Design review of the part built by this model. Coordinates are the model's own, in mm. A direction names the side the tool comes from. Give positions to 0.01 mm unless a question says otherwise; leave off trailing zeros. Write each loop counter-clockwise with the first axis right and the second up, starting at its lowest first coordinate (ties: lowest second). Pieces come first, ordered by that corner, then holes.
Autodesk Inventor part; units mm, degrees
ref_plane "YZ Plane" through (0, 0, 0) normal (1, 0, 0) x (0, 1, 0)
ref_plane "XZ Plane" through (0, 0, 0) normal (0, 1, 0) x (-1, 0, 0)
ref_plane "XY Plane" through (0, 0, 0) normal (0, 0, 1) x (1, 0, 0)
sketch "Sketch1" plane through (0, 0, 0) normal (0, 0, 1) x (1, 0, 0)
  line L0 (-30, -30) -> (30, -30)
  line L1 (30, -30) -> (30, 30)
  line L2 (30, 30) -> (-30, 30)
  line L3 (-30, 30) -> (-30, -30)
  line L4 (-30, -30) -> (30, 30) construction
  line L5 (30, -30) -> (-30, 30) construction
  point P0 (0, 0)
  dimension "d0" = 60
  dimension "d1" = 60
extrude "Main Block" add sketch "Sketch1" along normal blind 60
sketch "Sketch2" plane through (-30, 30, 0) normal (0, 1, 0) x (1, 0, 0)
  line L0 (0, -60) -> (60, -60) construction
  line L1 (0, 0) -> (60, 0) construction
  line L2 (60, -60) -> (0, 0) construction
  line L3 (51.25, -51.25) -> (8.75, -51.25)
  line L4 (8.75, -51.25) -> (8.75, -8.75)
  line L5 (8.75, -8.75) -> (51.25, -8.75)
  line L6 (51.25, -8.75) -> (51.25, -51.25)
  line L7 (51.25, -51.25) -> (8.75, -8.75) construction
  line L8 (8.75, -51.25) -> (51.25, -8.75) construction
  line L9 (30, -30) -> (30, -51.25) construction
  point P0 (30, 0)
  dimension "d4" = 42.5
  dimension "d5" = 42.5
extrude "Motor Void" cut sketch "Sketch2" against normal blind 58
sketch "Sketch3" plane through (-30, 30, 0) normal (0, 1, 0) x (1, 0, 0)
  line L0 (30, 0) -> (30, -8.75) construction
  line L1 (8.75, -8.75) -> (51.25, -8.75) construction
  line L2 (38.25, 0.125) -> (21.75, 0.125)
  line L3 (21.75, 0.125) -> (21.75, -8.875)
  line L4 (21.75, -8.875) -> (38.25, -8.875)
  line L5 (38.25, -8.875) -> (38.25, 0.125)
  line L6 (38.25, 0.125) -> (21.75, -8.875) construction
  line L7 (21.75, 0.125) -> (38.25, -8.875) construction
  point P0 (30, -4.375)
  dimension "d30" = 16.5
  dimension "d31" = 9
extrude "Cable Void" cut sketch "Sketch3" against normal blind 41
sketch "Sketch4" plane through (-30, -30, 0) normal (0, -1, 0) x (1, 0, 0)
  line L0 (0, 0) -> (0, 60) construction
  line L1 (60, 60) -> (0, 60) construction
  line L2 (0, 0) -> (60, 60) construction
  circle A0 centre (30, 30) radius 11
  point P0 (30, 0)
  dimension "d12" = 22
extrude "Raised Void" cut sketch "Sketch4" against normal blind 2
sketch "Sketch6" plane through (-30, -30, 0) normal (-1, 0, 0) x (0, 0, 1)
  line L0 (60, 0) -> (60, 60) construction
  line L1 (60, 60) -> (60, 55) construction
  line L2 (60, 55) -> (55, 55) construction
  line L3 (60, 0) -> (60, 5) construction
  line L4 (60, 5) -> (55, 5) construction
  line L5 (0, 0) -> (5, 0) construction
  line L6 (0, 0) -> (60, 0) construction
  line L7 (5, 0) -> (5, 5) construction
  line L8 (0, 60) -> (0, 0) construction
  line L9 (0, 60) -> (5, 60) construction
  line L10 (0, 60) -> (60, 60) construction
  line L11 (5, 60) -> (5, 55) construction
  circle A0 centre (55, 55) radius 1.5
  circle A1 centre (55, 5) radius 1.5
  circle A2 centre (5, 5) radius 1.5
  circle A3 centre (5, 55) radius 1.5
  point P0 (0, 30)
  dimension "d32" = 5
  dimension "d33" = 5
  dimension "d34" = 5
  dimension "d35" = 5
  dimension "d36" = 5
  dimension "d37" = 5
  dimension "d38" = 5
  dimension "d39" = 5
  dimension "d40" = 3
  dimension "d41" = 3
  dimension "d42" = 3
  dimension "d43" = 3
extrude "Holes" cut sketch "Sketch6" against normal blind 60
fillet "Cleaning it up" radius 5 5 edges at (0, 30, 60) (0, -30, 60) (19.125, 30, 0) (-19.125, 30, 0) (0, -30, 0)
equation "\"d4\" = d5"
properties part number "60x60Motor"
(1) Consider section D-D, the plane y = -4.5. Give the boundary of the cut face in (x, z).
Resolved:
outline: (-30, 0) - (-8.25, 0) - (-8.25, 8.75) - (-21.25, 8.75) - (-21.25, 51.25) - (21.25, 51.25) - (21.25, 8.75) - (8.25, 8.75) - (8.25, 0) - (30, 0) - (30, 60) - (-30, 60) - close
(2) Consider section A-A, the plane x = 19. Give the boundary of the cut face in (y, z).
Resolved:
outline: (-30, 5) arc R5 ccw to (-25, 0) - (25, 0) arc R5 ccw to (30, 5) - (30, 8.75) - (-28, 8.75) - (-28, 51.25) - (30, 51.25) - (30, 55) arc R5 ccw to (25, 60) - (-25, 60) arc R5 ccw to (-30, 55) - close; hole circle Ø3 at (-25, 5); hole circle Ø3 at (-25, 55); hole circle Ø3 at (25, 5); hole circle Ø3 at (25, 55)
(3) Mouldability with a two-part tool opening along Z and no side actions: class faces 1 (the face through (0, -11, 4)), 2 (the face through (-0.42, 26.265, 55.806)), 3 (the face through (-14, 0, 0)) as pulls with the +Z half, pulls with the -Z half, needs draft (parallel to the pull), parting line crosses it, or undercut.
Resolved:
face 1: needs draft
face 2: undercut
face 3: pulls with the -Z half
(4) Tool access review of faces 4 (the face through (-30, 0, 30)), 5 (the face through (8.25, 10, 4)), 6 (the face through (0, 1, 51.25)): name each direction out of +Z, -Z, +X, -X, +Y, -Y from which nothing blocks a thin tool from reaching the whole face with its end or side.
Resolved:
face 4: +Z, -Z, -X, +Y, -Y
face 5: -Z, +Y
face 6: +Y
(5) Consider section C-C, the plane z = 36.5. Give the boundary of the cut face in (x, y), then the cut area to 3 significant figures.
Resolved:
outline: (-30, -30) - (-8.87, -30) - (-8.87, -28) - (-21.25, -28) - (-21.25, 30) - (-30, 30) - close; (8.87, -30) - (30, -30) - (30, 30) - (21.25, 30) - (21.25, -28) - (8.87, -28) - close
area: 1,100 mm2
(6) To check wall thickness, follow L1, parallel to Y at x = 12, z = 55; L2, parallel to Z at x = -12, y = 15.5; L3, parallel to X at y = 4, z = 45. State the ranges of each line that lie inside material, in increasing order.
Resolved:
L1: y = -30 to -26.5, -23.5 to 23.5, 26.5 to 30
L2: z = 0 to 8.75, 51.25 to 60
L3: x = -30 to -21.25, 21.25 to 30
(7) Consider section B-B, the plane y = -22.5. Give the boundary of the cut face in (x, z).
Resolved:
outline: (-30, 0) - (30, 0) - (30, 60) - (-30, 60) - close; hole (-21.25, 8.75) - (21.25, 8.75) - (21.25, 51.25) - (-21.25, 51.25) - close
(8) Clearance check with flat-ended pins moving along their axes: P1, Ø2.5, axis at y = 25, z = 55, coming from the +X side; P2, Ø4, axis at x = 0, y = 11.5, coming from the -Z side; P3, Ø5, axis at x = 15, z = 44.5, coming from the +Y side; P4, Ø9.5, axis at x = -1.5, z = 3.5, coming from the +Y side. State where each tip first meets the part, or that it passes through.
Resolved:
P1: passes through
P2: stops at z = 51.25
P3: stops at y = -28
P4: stops at y = -11
